Model file for the job. Use its own axes, mm. Coordinates: 2 decimals unless noted, no trailing zeros. Write each loop counter-clockwise with the first axis right and the second up, starting at its lowest first coordinate (ties: lowest second). Pieces come first, ordered by that corner, then holes. Notation, with made-up numbers: M -18,-20.75 L 20,-20.75 A10 ccw 20,-15.75 Z; hole C -33.75,65.5 d4. An arc over 180 degrees is marked long. One line per question, with ' | ' between items. Start each with the question number.
(1) Flat gauge pins, fed straight in: pin 1 Ø3 at (x, y) = (138, 109.5) entering from -Z; pin 2 Ø10.5 at (x, y) = (40, 99.5) entering from +Z. Where does each tip first touch, or does it go through?
(2) Two-plate mould, pull along Y, no slides. Class faces 1 (the face through (30, 97, 15)), 2 (the face through (2.85, 3.01, 10.14)), 3 (the face through (183, 96, 10)): +Y half, -Y half, draft (parallel to the pull), parting line (faces both ways), or undercut.
(3) Cut at B-B (y = 38.5). Write the cut outline in (x, z).
(4) Wall check: probe 1 along X at (y, z) = (161.5, 14.75); probe 2 along Y at (x, z) = (43, 17.75); probe 3 along Z at (x, y) = (97.5, 34.5). Give the ranges that are in metal, low to high.
(5) Cut at A-A (x = 33.5). Write the cut outline in (y, z), plus the area to 3 significant figures.
from build123d import *

# Parameters (mm, degrees)
SKETCH1_W           = 183
SKETCH1_H           = 195
BOSS_EXTRUDE2_DEPTH = 20
SKETCH3_W           = 21
SKETCH3_H           = 25
CUT_EXTRUDE1_DEPTH  = 10
CUT_EXTRUDE2_DEPTH  = 135


with BuildPart() as part:
    # Sketch1 → Boss-Extrude2 (new body)
    with BuildSketch(Plane.XY):
        with Locations((91.5, 97.5)):
            Rectangle(SKETCH1_W, SKETCH1_H)
    extrude(amount=BOSS_EXTRUDE2_DEPTH)

    # Sketch3 → Cut-Extrude1 (cut)
    with BuildSketch(Plane.XY.offset(20)):
        with Locations((40.5, 97.5)):
            Rectangle(SKETCH3_W, SKETCH3_H)
        with Locations((40.5, 152.5)):
            Rectangle(SKETCH3_W, SKETCH3_H)
        with Locations((91.5, 152.5)):
            Rectangle(SKETCH3_W, SKETCH3_H)
        with Locations((40.5, 42.5)):
            Rectangle(SKETCH3_W, SKETCH3_H)
        with Locations((91.5, 97.5)):
            Rectangle(SKETCH3_W, SKETCH3_H)
        with Locations((91.5, 42.5)):
            Rectangle(SKETCH3_W, SKETCH3_H)
        with Locations((142.5, 97.5)):
            Rectangle(SKETCH3_W, SKETCH3_H)
        with Locations((142.5, 42.5)):
            Rectangle(SKETCH3_W, SKETCH3_H)
        with Locations((142.5, 152.5)):
            Rectangle(SKETCH3_W, SKETCH3_H)
    extrude(amount=-CUT_EXTRUDE1_DEPTH, mode=Mode.SUBTRACT)

    # Sketch4 → Cut-Extrude2 (cut)
    with BuildSketch(Plane.XY.offset(20)):
        with BuildLine():
            Line((0, 185), (0, 195))
            Line((0, 195), (10, 195))
            ThreePointArc((10, 195), (2.928932188, 192.071067812), (0, 185))
        make_face()
        with BuildLine():
            Line((173, 195), (183, 195))
            Line((183, 195), (183, 185))
            ThreePointArc((183, 185), (180.071067812, 192.071067812), (173, 195))
        make_face()
        with BuildLine():
            Line((183, 10), (183, 0))
            Line((183, 0), (173, 0))
            ThreePointArc((173, 0), (180.071067812, 2.928932188), (183, 10))
        make_face()
        with BuildLine():
            Line((10, 0), (0, 0))
            Line((0, 0), (0, 10))
            ThreePointArc((0, 10), (2.928932188, 2.928932188), (10, 0))
        make_face()
    extrude(amount=-CUT_EXTRUDE2_DEPTH, mode=Mode.SUBTRACT)


solid = part.part
Filled in:
1) pin 1: z = 0 | pin 2: z = 10
2) face 1: undercut | face 2: -Y half | face 3: draft
3) outline: M 0,0 L 183,0 L 183,20 L 153,20 L 153,10 L 132,10 L 132,20 L 102,20 L 102,10 L 81,10 L 81,20 L 51,20 L 51,10 L 30,10 L 30,20 L 0,20 Z
4) probe 1: 0 to 30, 51 to 81, 102 to 132, 153 to 183 | probe 2: 0 to 30, 55 to 85, 110 to 140, 165 to 195 | probe 3: 0 to 10
5) outline: M 0,0 L 195,0 L 195,20 L 165,20 L 165,10 L 140,10 L 140,20 L 110,20 L 110,10 L 85,10 L 85,20 L 55,20 L 55,10 L 30,10 L 30,20 L 0,20 Z | area: 3,150 mm²
